The listing builds one solid part. Answer for the finished solid, in the listing's coordinates (mm). Give positions to 0.01 mm unless a question says otherwise; leave off trailing zeros. Write each loop counter-clockwise with the first axis right and the second up, starting at its lowest first coordinate (ties: lowest second). Pieces come first, ordered by that corner, then holes. Notation, with made-up numbers: (75, 86) - (133, 86) arc R13 ccw to (133, 110) - close; hole circle Ø4 at (29, 60). An arc over 180 degrees is marked (long way). One line per question, with ' | ' between items. Start each with the question number.
1. A cutting plane is placed at A-A (x = 1481). Determine the outline of the cut face in (y, z).
2. Find the intervals of material crossed by L1, parallel to Z at x = 1704, y = -23.75; L2, parallel to Z at x = 1300, y = -17.75, in increasing order. Write a range as from..to.
3. Given P1, Ø12, axis at x = 800.5, y = -20.5, coming from the -Z side; P2, Ø10, axis at y = -5, z = 602, coming from the +X side (3 decimals), each flat-ended and moving along its own axis, determine where each tip first touches the part or whether it passes through.
4. A cutting plane is placed at B-B (z = 261.5). State how many separate pieces and enclosed holes the cut face has, then the cut area to 3 significant figures.
```python
from build123d import *

# Parameters (mm, degrees)
F0_W     = 12.7
F0_H     = 952.5
F1_DEPTH = 25.4


# Not quite as in the source:
# - a feature names something its author has since deleted; it is built from what else it names


with BuildPart() as f1:
    # F0 (on Front) → F1 (new body)
    with BuildSketch(Plane.XZ):
        Polygon((0, 1041.4), (0, 0), (101.6, 0), (101.6, 63.5), (101.6, 76.2), (101.6, 1028.7), (101.6, 1041.4), align=None)
        Polygon((101.6, 76.2), (101.6, 63.5), (2203.45, 63.5), (2203.45, 76.2), (2124.075, 76.2), (2111.375, 76.2), (2022.475, 76.2), (2009.775, 76.2), (1920.875, 76.2), (1908.175, 76.2), (1819.275, 76.2), (1806.575, 76.2), (1717.675, 76.2), (1704.975, 76.2), (1616.075, 76.2), (1603.375, 76.2), (1514.475, 76.2), (1501.775, 76.2), (1412.875, 76.2), (1400.175, 76.2), (1311.275, 76.2), (1298.575, 76.2), (1209.675, 76.2), (1196.975, 76.2), (1108.075, 76.2), (1095.375, 76.2), (1006.475, 76.2), (993.775, 76.2), (904.875, 76.2), (892.175, 76.2), (803.275, 76.2), (790.575, 76.2), (701.675, 76.2), (688.975, 76.2), (600.075, 76.2), (587.375, 76.2), (498.475, 76.2), (485.775, 76.2), (396.875, 76.2), (384.175, 76.2), (295.275, 76.2), (282.575, 76.2), (193.675, 76.2), (180.975, 76.2), align=None)
        with Locations((187.325, 552.45)):
            Rectangle(F0_W, F0_H)
        with Locations((288.925, 552.45)):
            Rectangle(F0_W, F0_H)
        with Locations((390.525, 552.45)):
            Rectangle(F0_W, F0_H)
        with Locations((492.125, 552.45)):
            Rectangle(F0_W, F0_H)
        with Locations((593.725, 552.45)):
            Rectangle(F0_W, F0_H)
        with Locations((695.325, 552.45)):
            Rectangle(F0_W, F0_H)
        with Locations((796.925, 552.45)):
            Rectangle(F0_W, F0_H)
        with Locations((898.525, 552.45)):
            Rectangle(F0_W, F0_H)
        with Locations((1000.125, 552.45)):
            Rectangle(F0_W, F0_H)
        with Locations((1101.725, 552.45)):
            Rectangle(F0_W, F0_H)
        with Locations((1203.325, 552.45)):
            Rectangle(F0_W, F0_H)
        with Locations((1304.925, 552.45)):
            Rectangle(F0_W, F0_H)
        with Locations((1406.525, 552.45)):
            Rectangle(F0_W, F0_H)
        with Locations((1508.125, 552.45)):
            Rectangle(F0_W, F0_H)
        with Locations((1609.725, 552.45)):
            Rectangle(F0_W, F0_H)
        with Locations((1711.325, 552.45)):
            Rectangle(F0_W, F0_H)
        with Locations((1812.925, 552.45)):
            Rectangle(F0_W, F0_H)
        with Locations((1914.525, 552.45)):
            Rectangle(F0_W, F0_H)
        Polygon((2203.45, 1041.4), (101.6, 1041.4), (101.6, 1028.7), (180.975, 1028.7), (193.675, 1028.7), (282.575, 1028.7), (295.275, 1028.7), (384.175, 1028.7), (396.875, 1028.7), (485.775, 1028.7), (498.475, 1028.7), (587.375, 1028.7), (600.075, 1028.7), (688.975, 1028.7), (701.675, 1028.7), (790.575, 1028.7), (803.275, 1028.7), (892.175, 1028.7), (904.875, 1028.7), (993.775, 1028.7), (1006.475, 1028.7), (1095.375, 1028.7), (1108.075, 1028.7), (1196.975, 1028.7), (1209.675, 1028.7), (1298.575, 1028.7), (1311.275, 1028.7), (1400.175, 1028.7), (1412.875, 1028.7), (1501.775, 1028.7), (1514.475, 1028.7), (1603.375, 1028.7), (1616.075, 1028.7), (1704.975, 1028.7), (1717.675, 1028.7), (1806.575, 1028.7), (1819.275, 1028.7), (1908.175, 1028.7), (1920.875, 1028.7), (2009.775, 1028.7), (2022.475, 1028.7), (2111.375, 1028.7), (2124.075, 1028.7), (2203.45, 1028.7), align=None)
        with Locations((2016.125, 552.45)):
            Rectangle(F0_W, F0_H)
        with Locations((2117.725, 552.45)):
            Rectangle(F0_W, F0_H)
    extrude(amount=F1_DEPTH)


solid = f1.part
```
Determined:
1) outline: (-25.4, 63.5) - (0, 63.5) - (0, 76.2) - (-25.4, 76.2) - close; (-25.4, 1028.7) - (0, 1028.7) - (0, 1041.4) - (-25.4, 1041.4) - close
2) L1: 63.5..76.2, 1028.7..1041.4 | L2: 63.5..1041.4
3) P1: z = 63.5 | P2: x = 2124.075
4) separate pieces: 21 | enclosed holes: 0 | area: 9,030 mm2
